Source: CAD feature listing. Evaluate the final solid. Frame: model axes, mm. Give positions to 0.01 mm unless a question says otherwise; leave off trailing zeros. Write each loop counter-clockwise with the first axis right and the second up, starting at its lowest first coordinate (ties: lowest second). Pieces come first, ordered by that corner, then holes. Notation, with made-up numbers: M -3.75,57.5 L 15.25,57.5 A19 ccw 15.25,94.5 Z; hole C -14,42.25 d10. An arc over 180 degrees is marked long. Answer as a JSON object with one key per item and string values. Group by question number.
```python
from build123d import *

# Parameters (mm, degrees)
F1_DEPTH = 30


# Not quite as in the source:
# - a feature of the source that left no trace in its solid (it failed there, or was rolled back) is left out
# - a feature names something its author has since deleted; it is built from what else it names


with BuildPart() as f1:
    # F0 (on Front) → F1 (new body)
    with BuildSketch(Plane.XZ):
        with BuildLine():
            ThreePointArc((-50.5958115044, -6.02955559), (-47.8576962726, -5.4409727065), (-45.0680997666, -5.1922637066))
            ThreePointArc((-45.0680997666, -5.1922637066), (-44.7014233398, 3.2450721847), (-47.4287139254, 11.2378798646))
            ThreePointArc((-47.4287139254, 11.2378798646), (-62.9262479802, 22.3973362627), (-81.478701042, 17.868151538))
            ThreePointArc((-81.478701042, 17.868151538), (-84.5846312596, 14.8818765302), (-87.0738165711, 11.3649748506))
            ThreePointArc((-87.0738165711, 11.3649748506), (-86.8766386462, -11.7015650942), (-66.6597911749, -22.8093651683))
            ThreePointArc((-66.6597911749, -22.8093651683), (-65.8563320665, -20.1264267988), (-64.7302441516, -17.5621275103))
            ThreePointArc((-64.7302441516, -17.5621275103), (-78.5071405294, 13.7509063134), (-50.5958115044, -6.02955559))
        make_face()
        with BuildLine():
            ThreePointArc((-47.4287139254, 11.2378798646), (-44.7014233398, 3.2450721847), (-45.0680997666, -5.1922637066))
            ThreePointArc((-45.0680997666, -5.1922637066), (-44.4403953733, -5.1836282573), (-43.8126909801, -5.1922637066))
            ThreePointArc((-43.8126909801, -5.1922637066), (-44.1262374484, 3.5955062023), (-41.0934242922, 11.8493087029))
            Line((-41.0934242922, 11.8493087029), (-41.0934242922, 59.9904626227))
            ThreePointArc((-41.0934242922, 59.9904626227), (-21.1129667901, 79.0608636102), (-1.7345135358, 59.3790337844))
            Line((-1.7345135358, 59.3790337844), (-1.7345135358, 11.2378798646))
            ThreePointArc((-1.7345135358, 11.2378798646), (-0.2806344187, 8.1505609331), (0.6965577317, 4.8809434977))
            ThreePointArc((0.6965577317, 4.8809434977), (1.6737498821, 8.1505609331), (3.1276289991, 11.2378798646))
            Line((3.1276289991, 11.2378798646), (3.1276289991, 45.9835585246))
            ThreePointArc((3.1276289991, 45.9835585246), (21.7197442499, 58.7768351813), (39.7009037986, 45.1381923457))
            Line((39.7009037986, 45.1381923457), (39.7009037986, 15.5334114315))
            ThreePointArc((39.7009037986, 15.5334114315), (42.9557629485, 11.0402047373), (45.0299754174, 5.8942687567))
            Line((45.0299754174, 5.8942687567), (45.0299754174, 45.9835585246))
            ThreePointArc((45.0299754174, 45.9835585246), (26.3569721709, 67.2830168196), (2.7973072292, 51.5575546089))
            Line((2.7973072292, 51.5575546089), (2.7973072292, 60.3419492483))
            ThreePointArc((2.7973072292, 60.3419492483), (-21.0300426798, 83.9928980167), (-44.5032843921, 59.9904626227))
            Line((-44.5032843921, 59.9904626227), (-44.5032843921, 49.1925225526))
            ThreePointArc((-44.5032843921, 49.1925225526), (-67.2766387272, 67.32921183), (-87.0738165711, 45.9835585246))
            Line((-87.0738165711, 45.9835585246), (-87.0738165711, 11.3649748506))
            ThreePointArc((-87.0738165711, 11.3649748506), (-84.5846312596, 14.8818765302), (-81.478701042, 17.868151538))
            Line((-81.478701042, 17.868151538), (-81.478701042, 45.8139192271))
            ThreePointArc((-81.478701042, 45.8139192271), (-64.5188702281, 58.9782000656), (-47.4287139254, 45.9835585246))
            Line((-47.4287139254, 45.9835585246), (-47.4287139254, 11.2378798646))
        make_face()
        with BuildLine():
            ThreePointArc((-43.8126909801, -5.1922637066), (-44.4403953733, -5.1836282573), (-45.0680997666, -5.1922637066))
            ThreePointArc((-45.0680997666, -5.1922637066), (-47.8576962726, -5.4409727065), (-50.5958115044, -6.02955559))
            ThreePointArc((-50.5958115044, -6.02955559), (-58.8656531806, -10.3218921863), (-64.7302441516, -17.5621275103))
            ThreePointArc((-64.7302441516, -17.5621275103), (-65.8563320665, -20.1264267988), (-66.6597911749, -22.8093651683))
            ThreePointArc((-66.6597911749, -22.8093651683), (-47.0537232386, -50.6694843019), (-21.6223947557, -28.001628875))
            ThreePointArc((-21.6223947557, -28.001628875), (-21.7725399464, -25.3883010097), (-22.2209995718, -22.8093651683))
            ThreePointArc((-22.2209995718, -22.8093651683), (-23.0778257417, -19.9827903731), (-24.2925817064, -17.2905711947))
            ThreePointArc((-24.2925817064, -17.2905711947), (-30.0151375661, -10.3218921863), (-37.9904438403, -6.1142060617))
            ThreePointArc((-37.9904438403, -6.1142060617), (-40.8716704219, -5.4644295279), (-43.8126909801, -5.1922637066))
        make_face()
        with BuildLine():
            ThreePointArc((-28.3212575169, -21.8035702343), (-27.4607721402, -24.8496563168), (-27.1706954296, -28.001628875))
            ThreePointArc((-27.1706954296, -28.001628875), (-47.5923679315, -44.9812521081), (-60.5595332298, -21.8035702343))
            ThreePointArc((-60.5595332298, -21.8035702343), (-55.3580861087, -14.6208006063), (-47.2776192349, -10.9665856726))
            ThreePointArc((-47.2776192349, -10.9665856726), (-44.4403953733, -10.7319289312), (-41.6031715118, -10.9665856726))
            ThreePointArc((-41.6031715118, -10.9665856726), (-33.522704638, -14.6208006063), (-28.3212575169, -21.8035702343))
        make_face(mode=Mode.SUBTRACT)
        with BuildLine():
            ThreePointArc((-17.209328187, -16.9419843412), (-20.7331119046, -17.4788467793), (-24.2925817064, -17.2905711947))
            ThreePointArc((-24.2925817064, -17.2905711947), (-23.0778257417, -19.9827903731), (-22.2209995718, -22.8093651683))
            ThreePointArc((-22.2209995718, -22.8093651683), (-21.0207224268, -22.8108156941), (-19.8220295884, -22.749148784))
            ThreePointArc((-19.8220295884, -22.749148784), (-18.7192509321, -19.7539774624), (-17.209328187, -16.9419843412))
        make_face()
        with BuildLine():
            ThreePointArc((0.318409666, -6.3669728281), (-2.8385741788, -6.8366801987), (-5.8991326911, -7.7423035215))
            ThreePointArc((-5.8991326911, -7.7423035215), (-12.3087515473, -11.4145268316), (-17.209328187, -16.9419843412))
            ThreePointArc((-17.209328187, -16.9419843412), (-18.7192509321, -19.7539774624), (-19.8220295884, -22.749148784))
            ThreePointArc((-19.8220295884, -22.749148784), (-1.125900704, -51.7064120801), (24.9076758738, -29.1161216121))
            ThreePointArc((24.9076758738, -29.1161216121), (24.6833038658, -25.92408489), (24.0146003931, -22.7948234918))
            ThreePointArc((24.0146003931, -22.7948234918), (23.0881839229, -20.1873038876), (21.8529406759, -17.7111011327))
            ThreePointArc((21.8529406759, -17.7111011327), (15.3942852462, -10.5783627076), (6.5696450929, -6.7422300764))
            ThreePointArc((6.5696450929, -6.7422300764), (3.8283507197, -6.3644588197), (1.0614855049, -6.3212981203))
            ThreePointArc((1.0614855049, -6.3212981203), (0.6897612956, -6.3411047495), (0.318409666, -6.3669728281))
        make_face()
        with BuildLine():
            ThreePointArc((19.3593751999, -29.1161216121), (-10.6177327064, -40.8107493967), (3.5207306993, -11.9058160812))
            ThreePointArc((3.5207306993, -11.9058160812), (12.1592087901, -15.0859031335), (17.936744923, -22.2522364789))
            ThreePointArc((17.936744923, -22.2522364789), (18.9999779483, -25.6112394448), (19.3593751999, -29.1161216121))
        make_face(mode=Mode.SUBTRACT)
        with BuildLine():
            ThreePointArc((3.1276289991, 11.2378798646), (1.6737498821, 8.1505609331), (0.6965577317, 4.8809434977))
            ThreePointArc((0.6965577317, 4.8809434977), (1.2247054391, 0), (0.6965577317, -4.8809434977))
            ThreePointArc((0.6965577317, -4.8809434977), (0.8672943666, -5.6040920216), (1.0614855049, -6.3212981203))
            ThreePointArc((1.0614855049, -6.3212981203), (3.8283507197, -6.3644588197), (6.5696450929, -6.7422300764))
            ThreePointArc((6.5696450929, -6.7422300764), (33.3344406342, 14.4182569257), (21.8529406759, -17.7111011327))
            ThreePointArc((21.8529406759, -17.7111011327), (23.0881839229, -20.1873038876), (24.0146003931, -22.7948234918))
            ThreePointArc((24.0146003931, -22.7948234918), (41.3940847955, -13.484015887), (45.0299754174, 5.8942687567))
            ThreePointArc((45.0299754174, 5.8942687567), (42.9557629485, 11.0402047373), (39.7009037986, 15.5334114315))
            ThreePointArc((39.7009037986, 15.5334114315), (20.3247315889, 22.6622288579), (3.1276289991, 11.2378798646))
        make_face()
    extrude(amount=F1_DEPTH)


solid = f1.part
```
(1) Ray query, L1, parallel to X at y = -14.75, z = 32; L2, parallel to X at y = -14.5, z = 0; L3, parallel to Z at x = -8, y = -7.5. Return the intervals inside material, ascending. Write a range as [from, to].
(2) Contact query for flat-ended pins moving along their axis: pin 1 Ø15 at (y, z) = (-18, 37) entering from -X; pin 2 Ø14 at (y, z) = (-11, 35.5) entering from +X; pin 3 Ø12 at (y, z) = (-9.5, 55) entering from -X; pin 4 Ø3 at (x, z) = (12, 54) entering from -Y. Output: stop coordinate, or through.
(3) Section D-D, the plane y = -22.25. State how many separate pieces and enclosed holes the cut face has, plus the area to 3 significant figures.
(4) Section B-B, the plane x = -55. Return loops of the section in (y, z).
(5) Section A-A, the plane z = 0. Return loops of the section in (x, y), plus the area to 3 significant figures.
(6) Section C-C, the plane z = 70. Return loops of the section in (x, y), plus the area to 3 significant figures.
(7) Pull-direction query (X, two-part tool) for faces 1 (the cylindrical face through (-44.145, -14.79, 3.473)), 2 (the flat face through (-43, -30, 11)), 3 (the flat face through (45.03, -15, 26)); classes: pulls with the +X half, pulls with the -X half, needs draft (parallel to the pull), parting line crosses it, or undercut.
Reported:
{
 "1": {"L1": "x = [-87.07, -81.48], [-47.43, -41.09], [-1.73, 3.13], [39.7, 45.03]", "L2": "x = [-90.11, -85.03], [-49.54, -44.41], [1.22, 5.24], [40.73, 45.8]", "L3": "z = [-49.58, -43.13], [-15.1, -8.65], [73.78, 80.2]"},
 "2": {"pin 1": "stops at x = -87.07", "pin 2": "stops at x = 45.03", "pin 3": "stops at x = -86.86", "pin 4": "passes through"},
 "3": {"separate pieces": "1", "enclosed holes": "7", "area": "4,430 mm2"},
 "4": {"outline": "M -30,-48.23 L 0,-48.23 L 0,-41.67 L -30,-41.67 Z; M -30,-14.34 L 0,-14.34 L 0,-7.77 L -30,-7.77 Z; M -30,12.81 L 0,12.81 L 0,19.23 L -30,19.23 Z; M -30,56.24 L 0,56.24 L 0,64.54 L -30,64.54 Z"},
 "5": {"outline": "M -90.11,-30 L -85.03,-30 L -85.03,0 L -90.11,0 Z; M -49.54,-30 L -44.41,-30 L -44.41,0 L -49.54,0 Z; M 1.22,-30 L 5.24,-30 L 5.24,0 L 1.22,0 Z; M 40.73,-30 L 45.8,-30 L 45.8,0 L 40.73,0 Z", "area": "579 mm2"},
 "6": {"outline": "M -42.44,-30 L -37.99,-30 L -37.99,0 L -42.44,0 Z; M -4.85,-30 L 0.74,-30 L 0.74,0 L -4.85,0 Z", "area": "301 mm2"},
 "7": {"face 1": "undercut", "face 2": "needs draft", "face 3": "pulls with the +X half"}
}
